For this review, take the finished solid that the model builds, in its own axes (mm). Face numbers are marked on the shaded views. A direction names the side the tool comes from. Coordinates: 2 decimals unless noted, no trailing zeros. Order: outer loops, then holes, each group sorted by start corner. A loop starts at its lowest first (then second) coordinate and runs counter-clockwise, first axis right, second up.
Autodesk Inventor part; units mm, degrees
ref_plane "YZ Plane" through (0, 0, 0) normal (1, 0, 0) x (0, 1, 0)
ref_plane "XZ Plane" through (0, 0, 0) normal (0, 1, 0) x (-1, 0, 0)
ref_plane "XY Plane" through (0, 0, 0) normal (0, 0, 1) x (1, 0, 0)
sketch "Sketch1" plane through (0, 0, 0) normal (0, 0, 1) x (1, 0, 0)
  line L0 (-490, 50) -> (490, 50)
  line L1 (490, 50) -> (490, 0)
  line L2 (490, 0) -> (-490, 0)
  line L3 (-490, 0) -> (-490, 50)
  point P0 (0, 0)
  point P1 (0, 0)
  dimension "d0" = 980
  dimension "d1" = 50
extrude "Plate1" add sketch "Sketch1" along normal blind 2
sketch "Sketch2" plane through (490, 2, 0) normal (0, -1, 0) x (1, 0, 0)
  line L0 (-980, 0) -> (0, 0)
  line L1 (0, 0) -> (0, 20)
  line L2 (0, 20) -> (-980, 20)
  line L3 (-980, 20) -> (-980, 0)
edge flange "Flange1" height 20 angle 90 thickness 2 bend radius 2.75 thickness toward (0, -1, 0) relief tear relief width 2 relief depth 1 edges at (0, 0, 2) wall of the first edge with corners at (-490, 2, 0) (490, 2, 0) (490, 2, 20) (-490, 2, 20)
bend "Bend1"
corner "Corner1"
sketch "Sketch5" plane through (0, 0, 0) normal (0, 0, -1) x (-1, 0, 0)
  line L0 (490, 50) -> (-490, 50)
  line L1 (490, 0) -> (-490, 0)
  circle A0 centre (0, 50) radius 30
  line L2 (-490, 0) -> (-490, 50)
  line L3 (490, 0) -> (490, 50)
  circle A1 centre (-490, 50) radius 30
  circle A2 centre (490, 50) radius 30
  line L4 (-246, 50) -> (-244, 50)
  line L5 (-244, 50) -> (-244, 19)
  line L6 (-244, 19) -> (-246, 19)
  line L7 (-246, 19) -> (-246, 50)
  line L8 (244, 50) -> (246, 50)
  line L9 (246, 50) -> (246, 19)
  line L10 (246, 19) -> (244, 19)
  line L11 (244, 19) -> (244, 50)
  line L12 (0, 50) -> (0, 0) construction
  point P0 (245, 19)
  point P1 (-245, 19)
  point P2 (-490, 20)
  point P3 (-460, 50)
  point P4 (-30, 50)
  point P5 (30, 50)
  point P6 (460, 50)
  point P7 (490, 20)
  point P8 (-244, 50)
  point P9 (246, 50)
  dimension "d33" = 60
  dimension "d34" = 2
  dimension "d35" = 31
  dimension "d36" = 490
extrude "Extrusion1" cut sketch "Sketch5" against normal through all contours L9 L10 L11 L0 | L0 L3 A2 | A0 L0 | L5 L6 L7 L0 | L2 L0 A1 picked at (470.2507, 47.7748) picked at (6.5355, 34.7298) picked at (-470.2507, 47.7748)
sketch "Sketch7" plane through (0, 0, 2) normal (0, 0, 1) x (1, 0, 0)
  line L0 (468.7934, 20.88) -> (468.7934, 8.88) construction
  line L1 (468.7934, 8.88) -> (280.354, 8.88) construction
  line L2 (280.354, 8.88) -> (280.354, 20.88) construction
  line L3 (280.354, 20.88) -> (468.7934, 20.88) construction
  line L4 (-244, 50) -> (-30, 50)
  point P0 (0, 0)
  point P1 (-1, 50)
  point P2 (1, 50)
  dimension "d30" = 12
mark "Mark1"
sketch "Sketch8" plane through (0, 0, 0) normal (0, 0, -1) x (-1, 0, 0)
  line L0 (-244, 50) -> (-51.6572, 50)
  line L1 (-51.6572, 50) -> (502.6857, 50)
  line L2 (502.6857, 50) -> (502.6857, -31.7842)
  line L3 (502.6857, -31.7842) -> (-51.6572, -31.7842)
  line L4 (-51.6572, -31.7842) -> (-51.6572, 50)
  point P0 (0, 0)
extrude "Extrusion3" cut sketch "Sketch8" along normal through all both and the other way through all
equation "\"d1\" = Стрингер_7"
equation "\"d2\" = Thickness"
equation "\"d3\" = BendReliefWidth"
equation "\"d4\" = BendReliefDepth"
equation "\"d5\" = MinimumRemnant"
equation "\"d6\" = TransitionRadius"
equation "\"d9\" = BendRadius"
equation "\"d10\" = CornerReliefSize"
equation "\"d11\" = GapSize"
equation "\"d12\" = JacobiRadiusSize"
equation "\"BendReliefWidth\" = Thickness"
equation "\"BendReliefDepth\" = 0.5 * Thickness"
equation "\"CornerReliefSize\" = 4 * Thickness"
equation "\"MinimumRemnant\" = 2 * Thickness"
equation "\"TransitionRadius\" = BendRadius"
equation "\"JacobiRadiusSize\" = BendRadius"
equation "\"GapSize\" = Thickness"
equation "\"Стрингер_7\" = 50"
properties part number "MSC 506 !!GNUT' ZERKAL'NO!!" material "Stainless Steel"
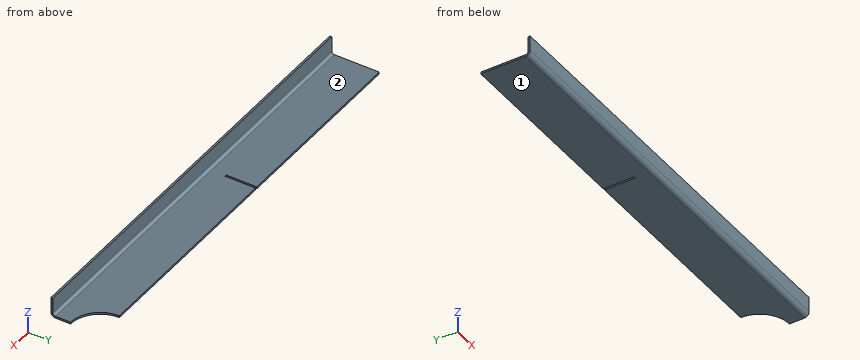
1. Take a section at C-C, the plane z = 17. Give the boundary of the cut face in (x, y).
Answer below:
outline: (51.66, 0) - (490, 0) - (490, 2) - (51.66, 2) - close
2. Take a section at B-B, the plane x = 253.5. Give the boundary of the cut face in (y, z), plus the area to 3 significant figures.
Answer below:
outline: (0, 4.75) arc R4.75 ccw to (4.75, 0) - (50, 0) - (50, 2) - (4.75, 2) arc R2.75 cw to (2, 4.75) - (2, 20) - (0, 20) - close
area: 133 mm2
3. Machinability: for the marked faces 1 and 2, which of the approach directions +Z, -Z, +X, -X, +Y, -Y give a long, thin tool a straight path to every point of the face, cutting with its end or side? Answer none if there is none.
Answer below:
face 1: -Z, +X, -X, +Y, -Y
face 2: +Z, +X, -X, +Y
4. To check wall thickness, follow L1, parallel to Y at x = 143, z = 10.5; L2, parallel to Y at x = 414, z = 3.75. State the ranges of each line that lie inside material, in increasing order.
Answer below:
L1: y = 0 to 2
L2: y = 0.11 to 2.19
5. Take a section at A-A, the plane y = 29. Give the boundary of the cut face in (x, z).
Answer below:
outline: (51.66, 0) - (244, 0) - (244, 2) - (51.66, 2) - close; (246, 0) - (468.58, 0) - (468.58, 2) - (246, 2) - close
6. Clearance check with flat-ended pins moving along their axes: pin 1 Ø4.5 at (x, z) = (267, 10.5) entering from +Y; pin 2 Ø1 at (y, z) = (30.5, 1.5) entering from +X; pin 3 Ø1 at (x, z) = (245, 1) entering from +Y. State where each tip first meets the part, or that it passes through.
Answer below:
pin 1: stops at y = 2
pin 2: stops at x = 467.64
pin 3: stops at y = 19
